```python
from build123d import *

# Parameters (mm, degrees)
SKETCH1_W               = 20
SKETCH1_H               = 22
BOSS_EXTRUDE1_DEPTH     = 16
SKETCH2_W               = 15
SKETCH2_H               = 5
CUT_EXTRUDE1_DEPTH      = 23
SKETCH3_R               = 3.96875
CUT_EXTRUDE2_DEPTH      = 13.875
CUT_EXTRUDE2_DEPTH_BACK = 4.125
CUT_EXTRUDE3_REACH      = 18
SKETCH4_R               = 4.7625
SKETCH5_R               = 5.762499999
SKETCH5_R_2             = 4.762499999
BOSS_EXTRUDE2_DEPTH     = 0.5
SKETCH6_R               = 5.2625
SKETCH6_R_2             = 3.96875
BOSS_EXTRUDE3_DEPTH     = 0.5
BOSS_EXTRUDE4_REACH     = 14.875
SKETCH7_W               = 15
SKETCH7_H               = 4
SKETCH9_R               = 1.5
CUT_EXTRUDE4_DEPTH      = 21


with BuildPart() as part:
    # Sketch1 → Boss-Extrude1 (new body)
    with BuildSketch(Plane(origin=(0, 0, 0), x_dir=(1, 0, 0), z_dir=(0, 1, 0))):
        with Locations((10, 11)):
            Rectangle(SKETCH1_W, SKETCH1_H)
    extrude(amount=BOSS_EXTRUDE1_DEPTH)

    # Sketch2 → Cut-Extrude1 (cut, through all)
    with BuildSketch(Plane(origin=(0, 0, -22), x_dir=(-1, 0, 0), z_dir=(0, 0, -1))):
        with Locations((-12.5, 5.625)):
            Rectangle(SKETCH2_W, SKETCH2_H)
    extrude(amount=-CUT_EXTRUDE1_DEPTH, mode=Mode.SUBTRACT)

    # Sketch3 → Cut-Extrude2 (cut, two sides)
    with BuildSketch(Plane(origin=(0, 3.125, 0), x_dir=(1, 0, 0), z_dir=(0, 1, 0))) as cut_extrude2_sk:
        with Locations((13.184494174, 13)):
            Circle(SKETCH3_R)
    extrude(amount=CUT_EXTRUDE2_DEPTH, mode=Mode.SUBTRACT)
    extrude(cut_extrude2_sk.sketch, amount=-CUT_EXTRUDE2_DEPTH_BACK, mode=Mode.SUBTRACT)

    # Sketch4 → Cut-Extrude3 (cut, up to next)
    with BuildSketch(Plane.XZ, mode=Mode.PRIVATE) as cut_extrude3_sk1:
        with Locations((13.184494174, -13)):
            Circle(SKETCH4_R)
    cut_extrude3_tool1 = extrude(cut_extrude3_sk1.sketch, amount=-CUT_EXTRUDE3_REACH, mode=Mode.PRIVATE) & part.part
    add(cut_extrude3_tool1.solids().sort_by_distance((13.184494, 0, -13))[0], mode=Mode.SUBTRACT)

    # Sketch5 → Boss-Extrude2 (add)
    with BuildSketch(Plane(origin=(0, 3.125, 0), x_dir=(1, 0, 0), z_dir=(0, 1, 0))):
        with Locations((13.184494174, 13)):
            Circle(SKETCH5_R)
        with Locations((13.184494174, 13)):
            Circle(SKETCH5_R_2, mode=Mode.SUBTRACT)
    extrude(amount=BOSS_EXTRUDE2_DEPTH)

    # Sketch6 → Boss-Extrude3 (add)
    with BuildSketch(Plane.XZ.offset(-8.125)):
        with Locations((13.184494174, -13)):
            Circle(SKETCH6_R)
        with Locations((13.184494174, -13)):
            Circle(SKETCH6_R_2, mode=Mode.SUBTRACT)
    extrude(amount=BOSS_EXTRUDE3_DEPTH)

    # Sketch7 → Boss-Extrude4 (add, up to next)
    with BuildSketch(Plane(origin=(0, 3.125, 0), x_dir=(1, 0, 0), z_dir=(0, 1, 0)), mode=Mode.PRIVATE) as boss_extrude4_sk1:
        with Locations((12.5, 2)):
            Rectangle(SKETCH7_W, SKETCH7_H)
    boss_extrude4_tool1 = extrude(boss_extrude4_sk1.sketch, amount=BOSS_EXTRUDE4_REACH, mode=Mode.PRIVATE) - part.part
    add(boss_extrude4_tool1.solids().sort_by_distance((12.5, 3.125, -2))[0])

    # Sketch9 → Cut-Extrude4 (cut, through all)
    with BuildSketch(Plane.ZY):
        with Locations((-3, 12)):
            Circle(SKETCH9_R)
        with Locations((-19, 12)):
            Circle(SKETCH9_R)
    extrude(amount=-CUT_EXTRUDE4_DEPTH, mode=Mode.SUBTRACT)


solid = part.part
```
Can you work these out from the model? Positions are in its coordinate system, mm. A direction names the side the tool comes from. Give positions to 0.01 mm unless a question says otherwise; leave off trailing zeros. Loops run counter-clockwise (first coordinate to the right, second up) from the corner with the lowest first, then second, coordinate; pieces in that order, holes last. Notation, with made-up numbers: M -15,20 L -5,20 A36 cw -5,58 Z; hole C 43,68 d5. An arc over 180 degrees is marked long. Use CSV: the item, a comma, the result in double quotes. Start each with the question number.
1. If I drill on L1, parallel to Y at x = 5.75, z = -15.75 (3 decimals); L2, parallel to Y at x = 17.25, z = -16.75 (3 decimals); L3, parallel to Y at x = 8.25, z = -18 (3 decimals), over which ranges is the centre line in solid material (lowest first)?
2. For P1, Ø1.5, axis at x = 14.5, y = 4.5, coming from the -Z side; P2, Ø2, axis at x = 16.5, y = 4.5, coming from the -Z side; P3, Ø2.5, axis at y = 4.5, z = -15, coming from the +X side, each with a flat end and sliding along its axis, tell me the tip position at first contact or that it passes through.
3. Imagine slicing it at C-C, the plane x = 10.25. Write out the boundary of the cut face in (y, z) (3 decimals).
4. Imagine slicing it at B-B, the plane z = -3. Write out the boundary of the cut face in (x, y).
5. On a 3-axis mill with a long thin cutter (end or side, diameter ignored), from which of +Z, -Z, +X, -X, +Y, -Y can I reach the whole of each face in a straight line? I mean faces 1 (the face through (18.204, 7.878, -11.419)), 2 (the face through (5, 6, -13)), 3 (the face through (12, 6, -4)). Say none if no direction works.
6. If we mould it in two halves opening along Y, with no side actions, what happens to faces 4 (the face through (8, 16, -11)), 5 (the face through (9.86, 12.07, -20.5)), 6 (the face through (20, 10, -11))? For each: released by +Y, released by -Y, zero draft, split by the parting line, or undercut.
7. Imagine slicing it at D-D, the plane z = -13. Write out the boundary of the cut face in (x, y) (3 decimals), plus the area to 3 significant figures.
8. Imagine slicing it at A-A, the plane y = 12. Write out the boundary of the cut face in (x, z).
Response values:
1,L1,"0 to 3.125, 8.125 to 16"
1,L2,"0 to 3.625, 8.125 to 16"
1,L3,"0 to 3.125, 8.125 to 10.882, 13.118 to 16"
2,P1,"z = -4"
2,P2,"z = -18.02"
2,P3,"x = 18.84"
3,outline,"M 0,-22 L 3.125,-22 L 3.125,-17.959 L 3.625,-17.959 L 3.625,-16.751 L 0,-16.751 Z; M 0,-9.249 L 3.625,-9.249 L 3.625,-8.041 L 3.125,-8.041 L 3.125,-4 L 8.125,-4 L 8.125,-8.632 L 7.625,-8.632 L 7.625,-10.328 L 16,-10.328 L 16,0 L 0,0 Z; M 7.625,-17.368 L 8.125,-17.368 L 8.125,-22 L 16,-22 L 16,-15.672 L 7.625,-15.672 Z; hole C 12,-19 d3; hole C 12,-3 d3"
4,outline,"M 0,0 L 20,0 L 20,10.5 L 0,10.5 Z; M 0,13.5 L 20,13.5 L 20,16 L 0,16 Z"
5,face 1,"none"
5,face 2,"-Z"
5,face 3,"+X"
6,face 4,"released by +Y"
6,face 5,"undercut"
6,face 6,"zero draft"
7,outline,"M 0,0 L 8.422,0 L 8.422,3.625 L 7.422,3.625 L 7.422,3.125 L 5,3.125 L 5,8.125 L 7.922,8.125 L 7.922,7.625 L 9.216,7.625 L 9.216,16 L 0,16 Z; M 17.153,7.625 L 18.447,7.625 L 18.447,8.125 L 20,8.125 L 20,16 L 17.153,16 Z; M 17.947,0 L 20,0 L 20,3.125 L 18.947,3.125 L 18.947,3.625 L 17.947,3.625 Z"
7,area,"155 mm^2"
8,outline,"M 0,-22 L 20,-22 L 20,-20.5 L 0,-20.5 Z; M 0,-17.5 L 20,-17.5 L 20,-4.5 L 0,-4.5 Z; M 0,-1.5 L 20,-1.5 L 20,0 L 0,0 Z; hole C 13.18,-13 d7.94"
